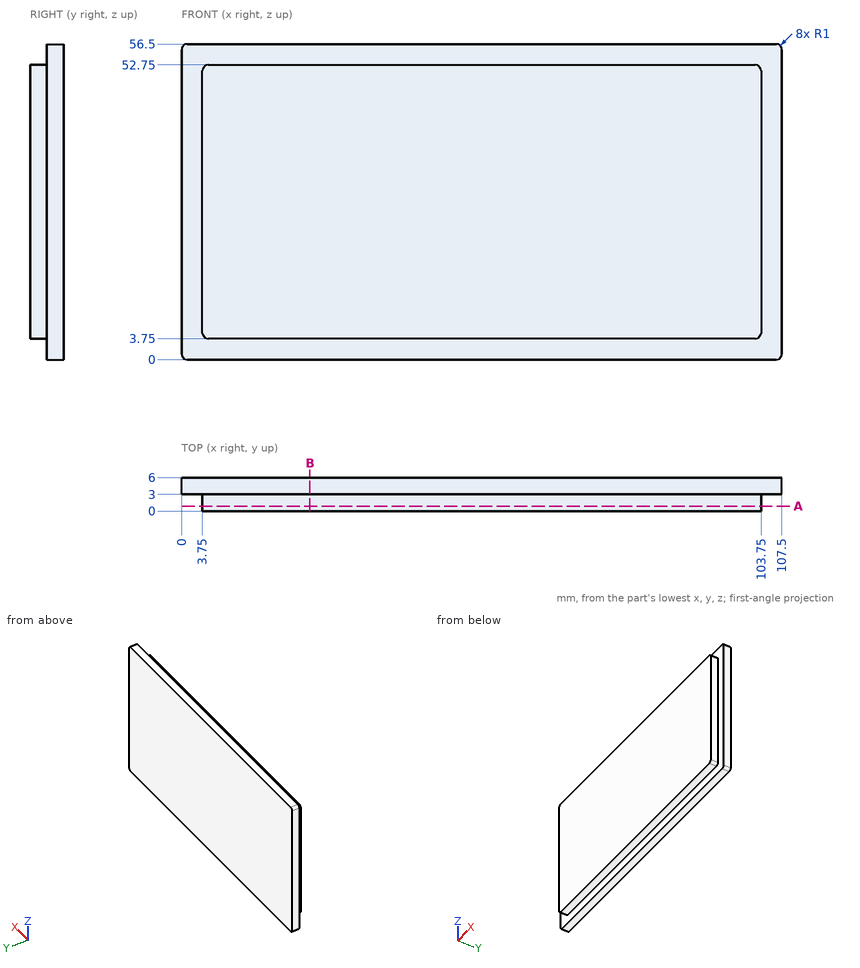
Print and shaded views of the part. All mm, measured from the part's lowest x, y and z. Round coordinates to 2 decimals unless told otherwise and drop trailing zeros. Order: outer loops, then holes, each group sorted by start corner. A loop starts at its lowest first (then second) coordinate and runs counter-clockwise, first axis right, second up. Notation, with made-up numbers: (-17, 49) - (27, 49) arc R26 cw to (27, 86) - close; hole circle Ø4 at (0, 56.5). An arc over 180 degrees is marked (long way). Use a Markdown table: item, result.
1) Flat gauge pins, fed straight in: pin 1 Ø1.5 at (y, z) = (2, 33) entering from -X; pin 2 Ø0.9 at (y, z) = (2, 26.5) entering from +X. Where does each tip first touch, or does it go through?
Recorded:
| item | result |
|---|---|
| pin 1 | stops at x = 3.75 |
| pin 2 | stops at x = 103.75 |
2) Wall check: L1, parallel to X at y = 1.45, z = 41; L2, parallel to Z at x = 37.5, y = 1.35; L3, parallel to Y at x = 48.5, z = 53. Give the ranges that are in metal, low to high.
Recorded:
| item | result |
|---|---|
| L1 | x = 3.75 to 103.75 |
| L2 | z = 3.75 to 52.75 |
| L3 | y = 3 to 6 |
3) Saw through at B-B on x = 23. Write the cut outline in (y, z).
Recorded:
| item | result |
|---|---|
| outline | (0, 3.75) - (3, 3.75) - (3, 0) - (6, 0) - (6, 56.5) - (3, 56.5) - (3, 52.75) - (0, 52.75) - close |
4) Saw through at A-A on y = 0.9. Write the cut outline in (x, z), and give its area (3 significant figures).
Recorded:
| item | result |
|---|---|
| outline | (3.75, 4.75) arc R1 ccw to (4.75, 3.75) - (102.75, 3.75) arc R1 ccw to (103.75, 4.75) - (103.75, 51.75) arc R1 ccw to (102.75, 52.75) - (4.75, 52.75) arc R1 ccw to (3.75, 51.75) - close |
| area | 4,900 mm² |
